Could you check a few things on this model? Use its own coordinates, in mm. Face numbers are marked on the shaded views. A direction names the side the tool comes from. Give positions to 0.01 mm unless a question says otherwise; leave off trailing zeros. Order: outer loops, then holes, each group sorted by start corner. A loop starts at its lowest first (then second) coordinate and runs counter-clockwise, first axis right, second up. Notation, with made-up numbers: (-9.75, 0.5) -> (3.25, 0.5) arc R21 cw to (3.25, 13.5) -> close; hole circle Ø6 at (63, 65.25). An arc over 180 degrees is marked (long way). One line per item, written item: value.
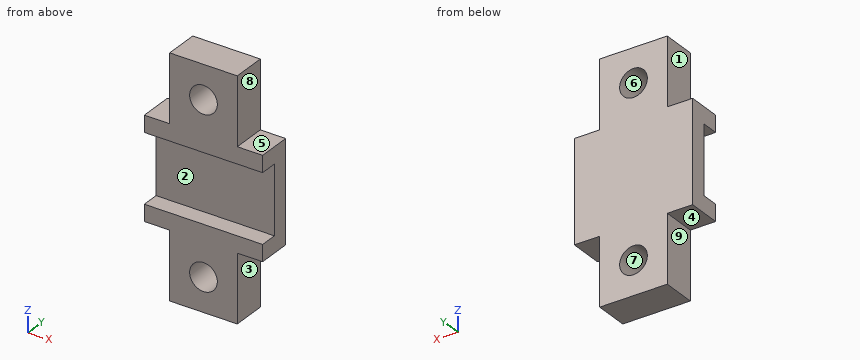
```python
from build123d import *

# Parameters (mm, degrees)
SKETCH1_W                = 20
SKETCH1_H                = 70
BOSS_EXTRUDE1_DEPTH      = 10
CUT_EXTRUDE1_DEPTH       = 42.533119315
CUT_EXTRUDE1_DEPTH_BACK  = 42.533119315
SKETCH2_W                = 20.25
SKETCH2_H                = 5.1
SKETCH3_R                = 4.1
CUT_EXTRUDE2_DEPTH       = 38.749172176
BOSS_EXTRUDE2_DEPTH      = 7.5
BOSS_EXTRUDE2_DEPTH_BACK = 27.5


with BuildPart() as part:
    # Sketch1 → Boss-Extrude1 (new body)
    with BuildSketch(Plane(origin=(0, 0, 0), x_dir=(1, 0, 0), z_dir=(0, 1, 0))):
        Rectangle(SKETCH1_W, SKETCH1_H)
    extrude(amount=BOSS_EXTRUDE1_DEPTH)

    # Sketch2 → Cut-Extrude1 (cut, two sides: drawn at the far end of the back side and taken through both)
    with BuildSketch(Plane(origin=(10, 0, 0), x_dir=(0, 0, -1), z_dir=(1, 0, 0)).offset(-CUT_EXTRUDE1_DEPTH_BACK)):
        with Locations((0, 2.55)):
            Rectangle(SKETCH2_W, SKETCH2_H)
    extrude(amount=CUT_EXTRUDE1_DEPTH + CUT_EXTRUDE1_DEPTH_BACK, mode=Mode.SUBTRACT)

    # Sketch3 → Cut-Extrude2 (cut, through all)
    with BuildSketch(Plane.XZ):
        with Locations(Location((0, 25, 0), (0, 0, 270))):
            Circle(SKETCH3_R)
        with Locations(Location((0, -25, 0), (0, 0, 270))):
            Circle(SKETCH3_R)
    extrude(amount=-CUT_EXTRUDE2_DEPTH, mode=Mode.SUBTRACT)

    # Sketch4 → Boss-Extrude2 (add, two sides: drawn at the far end of the back side and taken through both)
    with BuildSketch(Plane(origin=(10, 0, 0), x_dir=(0, 0, -1), z_dir=(1, 0, 0)).offset(-BOSS_EXTRUDE2_DEPTH_BACK)):
        Polygon((-10.125, 0), (-15.005, 0), (-15.005, 10), (15.005, 10), (15.005, 0), (10.125, 0), (10.125, 5.1), (-10.125, 5.1), align=None)
    extrude(amount=BOSS_EXTRUDE2_DEPTH + BOSS_EXTRUDE2_DEPTH_BACK)


solid = part.part
```
1) For the marked faces 1, 2, 3, 4 and 5, which set-ups out of +Z, -Z, +X, -X, +Y, -Y let a thin tool reach every point of the face, with its end or its side?
Answer below:
face 1: +Z, -X, +Y, -Y
face 2: +X, -X, -Y
face 3: -Z, +X, +Y, -Y
face 4: -Z, -X, +Y, -Y
face 5: +Z, +X, +Y, -Y
2) Suppose I cut it at B-B, the plane z = 25. Write out the boundary of the cut face in (x, y).
Answer below:
outline: (-10, 0) -> (-4.1, 0) -> (-4.1, 10) -> (-10, 10) -> close; (4.1, 0) -> (10, 0) -> (10, 10) -> (4.1, 10) -> close
3) Suppose I cut it at A-A, the plane y = 3. Write out the boundary of the cut face in (x, z) (3 decimals), then the cut area to 3 significant figures.
Answer below:
outline: (-17.5, -15.005) -> (-10, -15.005) -> (-10, -35) -> (10, -35) -> (10, -15.005) -> (17.5, -15.005) -> (17.5, -10.125) -> (-17.5, -10.125) -> close; (-17.5, 10.125) -> (17.5, 10.125) -> (17.5, 15.005) -> (10, 15.005) -> (10, 35) -> (-10, 35) -> (-10, 15.005) -> (-17.5, 15.005) -> close; hole circle Ø8.2 at (0, -25); hole circle Ø8.2 at (0, 25)
area: 1,040 mm2
4) If I drill on line 1 along X through (y, z) = (7, 25); line 2 along Z through (x, y) = (3.5, 7.5); line 3 along Y through (x, z) = (15, 9), over which ranges is the centre line in solid material (lowest first)?
Answer below:
line 1: x = -10 to -4.1, 4.1 to 10
line 2: z = -35 to -27.14, -22.86 to 22.86, 27.14 to 35
line 3: y = 5.1 to 10
5) Suppose I cut it at D-D, the plane y = 7. Write out the boundary of the cut face in (x, z) (3 decimals).
Answer below:
outline: (-17.5, -15.005) -> (-10, -15.005) -> (-10, -35) -> (10, -35) -> (10, -15.005) -> (17.5, -15.005) -> (17.5, 15.005) -> (10, 15.005) -> (10, 35) -> (-10, 35) -> (-10, 15.005) -> (-17.5, 15.005) -> close; hole circle Ø8.2 at (0, -25); hole circle Ø8.2 at (0, 25)
6) For P1, Ø4, axis at y = 1.5, z = -24.5, coming from the +X side; P2, Ø3, axis at y = 5.5, z = 23, coming from the -X side; P3, Ø4, axis at x = -14, y = 5, coming from the +Z side (3 decimals), each with a flat end and sliding along its axis, tell me the tip position at first contact or that it passes through.
Answer below:
P1: stops at x = 10
P2: stops at x = -10
P3: stops at z = 15.005
7) We'd pull the mould along X, two halves only. Please class the marked faces 6, 7, 8 and 9: +X half, -X half, draft (parallel to the pull), parting line (faces both ways), or undercut.
Answer below:
face 6: undercut
face 7: undercut
face 8: +X half
face 9: -X half
8) Suppose I cut it at C-C, the plane x = 0. Write out the boundary of the cut face in (y, z) (3 decimals).
Answer below:
outline: (0, -35) -> (10, -35) -> (10, -29.1) -> (0, -29.1) -> close; (0, -20.9) -> (10, -20.9) -> (10, 20.9) -> (0, 20.9) -> (0, 10.125) -> (5.1, 10.125) -> (5.1, -10.125) -> (0, -10.125) -> close; (0, 29.1) -> (10, 29.1) -> (10, 35) -> (0, 35) -> close
